Geometry check sheet. Reference: the model listing, model coordinates, mm. A direction names the side the tool comes from. Coordinates: 2 decimals unless noted, no trailing zeros. Loops run counter-clockwise (first coordinate to the right, second up) from the corner with the lowest first, then second, coordinate; pieces in that order, holes last.
from build123d import *

# Parameters (mm, degrees)
ESQUISSE1_W             = 82.2
ESQUISSE1_H             = 20
BOSS_EXTRU_1_DEPTH      = 30
ENL_V_MAT_EXTRU_1_DEPTH = 3
CONG_1_R                = 5
CONG_2_R                = 0.5
ESQUISSE8_R             = 2.103774153
ENL_V_MAT_EXTRU_3_DEPTH = 90.759901961


with BuildPart() as part:
    # Esquisse1 → Boss.-Extru.1 (new body)
    with BuildSketch(Plane.XY):
        with Locations((-41.1, 10)):
            Rectangle(ESQUISSE1_W, ESQUISSE1_H)
    extrude(amount=BOSS_EXTRU_1_DEPTH)

    # Esquisse2 → Enlèv. mat.-Extru.1 (cut)
    with BuildSketch(Plane.XY.offset(30)):
        Polygon((-41.1, 5.4966679), (-37.2, 7.74833395), (-37.2, 12.25166605), (-41.1, 14.5033321), (-45, 12.25166605), (-45, 7.74833395), align=None)
    extrude(amount=-ENL_V_MAT_EXTRU_1_DEPTH, mode=Mode.SUBTRACT)

    # Congé1
    cong_1_edges = [part.edges().sort_by_distance(p)[0] for p in [
        (0, 0, 15),
        (-82.2, 0, 15),
        (-82.2, 20, 15),
        (0, 20, 15),
    ]]
    fillet(cong_1_edges, radius=CONG_1_R)

    # Congé2
    cong_2_edges = [part.edges().sort_by_distance(p)[0] for p in [
        (-43.05, 6.622500925, 30),
        (-39.15, 6.622500925, 30),
        (-37.2, 10, 30),
        (-39.15, 13.377499075, 30),
        (-43.05, 13.377499075, 30),
        (-45, 10, 30),
    ]]
    fillet(cong_2_edges, radius=CONG_2_R)

    # Esquisse8 → Enlèv. mat.-Extru.3 (cut, through all)
    with BuildSketch(Plane.XY):
        with Locations((-41.1, 10)):
            Circle(ESQUISSE8_R)
    extrude(amount=ENL_V_MAT_EXTRU_3_DEPTH, mode=Mode.SUBTRACT)


solid = part.part
1) Depth check by flat-ended pin: pin 1 (6.5 mm diameter, centred on x = -41.1, y = 10, fed in from -Z). Enter the tip coordinate at first touch or a pass-through.
Data:
pin 1: stops at z = 0
2) Section check C-C on y = 17.5. Record the cut outline in (x, z), and give its area (3 significant figures).
Data:
outline: (-81.53, 0) - (-0.67, 0) - (-0.67, 30) - (-81.53, 30) - close
area: 2,430 mm2
3) Material ranges on probe 1 along X at (y, z) = (10, 21.5); probe 2 along Y at (x, z) = (-41.1, 13.75); probe 3 along Y at (x, z) = (-78.5, 14), recorded low to high.
Data:
probe 1: x = -82.2 to -43.2, -39 to 0
probe 2: y = 0 to 7.9, 12.1 to 20
probe 3: y = 0.17 to 19.83
4) Section check B-B on z = 14.5. Record the cut outline in (x, y).
Data:
outline: (-82.2, 5) arc R5 ccw to (-77.2, 0) - (-5, 0) arc R5 ccw to (0, 5) - (0, 15) arc R5 ccw to (-5, 20) - (-77.2, 20) arc R5 ccw to (-82.2, 15) - close; hole circle Ø4.21 at (-41.1, 10)
5) Mould release check, pull along Y, two halves, no side actions. Record for faces 3 (the cylindrical face through (-2, 19, 15)), 4 (the flat face through (-43.08, 6.64, 28.27)), 5 (the flat face through (-42, 17, 30)): +Y half, -Y half, draft (parallel to the pull), parting line (faces both ways), or undercut.
Data:
face 3: +Y half
face 4: undercut
face 5: draft
6) Section check A-A on y = 10. Record the cut outline in (x, z).
Data:
outline: (-82.2, 0) - (-43.2, 0) - (-43.2, 27) - (-45, 27) - (-45, 29.5) arc R0.5 ccw to (-45.5, 30) - (-82.2, 30) - close; (-39, 0) - (0, 0) - (0, 30) - (-36.7, 30) arc R0.5 ccw to (-37.2, 29.5) - (-37.2, 27) - (-39, 27) - close
7) Access from +Z, -Z, +X, -X, +Y, -Y to the whole of each face (thin tool, end or side, straight path). Record for faces 1 (the cylindrical face through (-80.77, 1.5, 15.21)), 2 (the flat face through (-39.12, 13.36, 28.27)).
Data:
face 1: +Z, -Z, -X, -Y
face 2: +Z
